```python
from build123d import *

# Parameters (mm, degrees)
SHOULDER_DEPTH               = 20
SHELL_T                      = -4
SKETCH2_R                    = 2.4
PIVOT_HOLES_DEPTH            = 49.218253805
BASE_MOUNT_REACH             = 43.533
SKETCH4_R                    = 2.4
BASE_MOUNT_DIRECTION_2_DEPTH = 42.533119315


with BuildPart() as part:
    # Sketch1 → shoulder (new, symmetric)
    with BuildSketch(Plane(origin=(0, 0, 0), x_dir=(0, 0, -1), z_dir=(1, 0, 0))):
        with BuildLine():
            Line((10, 0), (10, -25))
            Line((10, -25), (-10, -25))
            Line((-10, -25), (-10, 0))
            ThreePointArc((-10, 0), (0, 10), (10, 0))
        make_face()
    extrude(amount=SHOULDER_DEPTH, both=True)

    # shell
    shell_openings = [part.faces().sort_by_distance(p)[0] for p in [
        (0, -12.5, -10),
        (0, -12.5, 10),
        (0, 10, 0),
    ]]
    offset(amount=SHELL_T, openings=shell_openings, kind=Kind.INTERSECTION)

    # Sketch2 → pivot holes (cut, through all)
    with BuildSketch(Plane(origin=(20, 0, 0), x_dir=(0, 0, -1), z_dir=(1, 0, 0))):
        Circle(SKETCH2_R)
    extrude(amount=-PIVOT_HOLES_DEPTH, mode=Mode.SUBTRACT)

    # Sketch4 → base mount (cut, up to next)
    with BuildSketch(Plane.XZ.offset(25), mode=Mode.PRIVATE) as base_mount_sk1:
        with Locations(Location((0, 0, 0), (0, 0, 90))):
            Circle(SKETCH4_R)
    base_mount_tool1 = extrude(base_mount_sk1.sketch, amount=-BASE_MOUNT_REACH, mode=Mode.PRIVATE) & part.part
    add(base_mount_tool1.solids().sort_by_distance((0, -25, 0))[0], mode=Mode.SUBTRACT)

    # Sketch4 → base mount direction 2 (cut)
    with BuildSketch(Plane.XZ.offset(25)):
        with Locations(Location((0, 0, 0), (0, 0, 90))):
            Circle(SKETCH4_R)
    extrude(amount=BASE_MOUNT_DIRECTION_2_DEPTH, mode=Mode.SUBTRACT)


solid = part.part
```
Geometry check sheet. Reference: the model listing, model coordinates, mm. A direction names the side the tool comes from. Give positions to 0.01 mm unless a question says otherwise; leave off trailing zeros. Write each loop counter-clockwise with the first axis right and the second up, starting at its lowest first coordinate (ties: lowest second). Pieces come first, ordered by that corner, then holes. Notation, with made-up numbers: (43, 70.25) -> (60, 70.25) arc R15 ccw to (60, 75.25) -> close; hole circle Ø7 at (2.25, 7.25). An arc over 180 degrees is marked (long way). Use one line per item in the form item = value.
Item 1: Sectioned sample at C-C on x = 0. Enter the section's corners in (y, z).
Results list:
outline = (-25, -10) -> (-21, -10) -> (-21, -2.4) -> (-25, -2.4) -> close; (-25, 2.4) -> (-21, 2.4) -> (-21, 10) -> (-25, 10) -> close
Item 2: Access from +Z, -Z, +X, -X, +Y, -Y to the whole of each face (thin tool, end or side, straight path). Record for faces 1 (the cylindrical face through (18.028, 2.024, -1.29)), 2 (the flat face through (4, -21, 0)).
Results list:
face_1 = +X, -X
face_2 = +Z, -Z, +Y
Item 3: Sectioned sample at A-A on z = 0. Enter the section's corners in (x, y).
Results list:
outline = (-20, -25) -> (-2.4, -25) -> (-2.4, -21) -> (-16, -21) -> (-16, -2.4) -> (-20, -2.4) -> close; (-20, 2.4) -> (-16, 2.4) -> (-16, 10) -> (-20, 10) -> close; (2.4, -25) -> (20, -25) -> (20, -2.4) -> (16, -2.4) -> (16, -21) -> (2.4, -21) -> close; (16, 2.4) -> (20, 2.4) -> (20, 10) -> (16, 10) -> close
Item 4: Scan lines: line 1 (X direction, y = -12.5, z = 6.75); line 2 (Y direction, x = 17.8, z = 0); line 3 (X direction, y = -23.6, z = 0). Record each from-to range of solid material in increasing order.
Results list:
line_1 = -20 to -16, 16 to 20
line_2 = -25 to -2.4, 2.4 to 10
line_3 = -20 to -2.4, 2.4 to 20
Item 5: Mould release check, pull along X, two halves, no side actions. Record for faces 3 (the flat face through (-20, -7, 0)), 4 (the flat face through (20, -7, 0)), 5 (the flat face through (0, -22, -10)), 6 (the flat face through (-16, -5, 0)): released by +X, released by -X, zero draft, split by the parting line, or undercut.
Results list:
face_3 = released by -X
face_4 = released by +X
face_5 = zero draft
face_6 = undercut
Item 6: Sectioned sample at B-B on y = -3. Enter the section's corners in (x, z), plus the area to 3 significant figures.
Results list:
outline = (-20, -10) -> (-16, -10) -> (-16, 10) -> (-20, 10) -> close; (16, -10) -> (20, -10) -> (20, 10) -> (16, 10) -> close
area = 160 mm2
Item 7: Depth check by flat-ended pin: pin 1 Ø3 at (x, z) = (0, 0) entering from -Y; pin 2 Ø6 at (x, z) = (-5, -0.5) entering from +Y. Enter the tip coordinate at first touch or a pass-through.
Results list:
pin_1 = through
pin_2 = -21
Item 8: Sectioned sample at D-D on x = -12.5. Enter the section's corners in (y, z).
Results list:
outline = (-25, -10) -> (-21, -10) -> (-21, 10) -> (-25, 10) -> close
